from build123d import *

# Parameters (mm, degrees)
SKETCH1_W                = 65
SKETCH1_H                = 51.3
BOSS_EXTRUDE1_DEPTH      = 1.5
SKETCH2_W                = 17.929597568
SKETCH2_H                = 18
BOSS_EXTRUDE2_DEPTH      = 1
BOSS_EXTRUDE3_DEPTH      = 9
BOSS_EXTRUDE3_DEPTH_BACK = 11
SKETCH4_W                = 61
SKETCH4_H                = 3.022614149
SKETCH5_W                = 65
SKETCH5_H                = 51.3
BOSS_EXTRUDE4_DEPTH      = 1.5


with BuildPart() as part:
    # Sketch1 → Boss-Extrude1 (new body)
    with BuildSketch(Plane(origin=(0, 0, 0), x_dir=(1, 0, 0), z_dir=(0, 1, 0))):
        Rectangle(SKETCH1_W, SKETCH1_H)
    extrude(amount=BOSS_EXTRUDE1_DEPTH)

    # Sketch2 → Boss-Extrude2 (add)
    with BuildSketch(Plane(origin=(0, 1.5, 0), x_dir=(1, 0, 0), z_dir=(0, 1, 0))):
        with Locations((0, 11.65)):
            Rectangle(SKETCH2_W, SKETCH2_H)
        with Locations((0, -11.65)):
            Rectangle(SKETCH2_W, SKETCH2_H)
    extrude(amount=BOSS_EXTRUDE2_DEPTH)

    # Sketch4 → Boss-Extrude3 (add, two sides: drawn at the far end of the back side and taken through both)
    with BuildSketch(Plane.XZ.offset(-BOSS_EXTRUDE3_DEPTH_BACK)):
        with Locations((0, 22.138692926)):
            Rectangle(SKETCH4_W, SKETCH4_H)
        with Locations((0, -22.138692926)):
            Rectangle(SKETCH4_W, SKETCH4_H)
    extrude(amount=BOSS_EXTRUDE3_DEPTH + BOSS_EXTRUDE3_DEPTH_BACK)

    # Sketch5 → Boss-Extrude4 (add)
    with BuildSketch(Plane.XZ.offset(9)):
        Rectangle(SKETCH5_W, SKETCH5_H)
    extrude(amount=BOSS_EXTRUDE4_DEPTH)


solid = part.part
Geometry check sheet. Reference: the model listing, model coordinates, mm. A direction names the side the tool comes from. Round coordinates to 2 decimals unless told otherwise and drop trailing zeros. Loops run counter-clockwise (first coordinate to the right, second up) from the corner with the lowest first, then second, coordinate; pieces in that order, holes last. Notation, with made-up numbers: (86, -9) -> (102, -9) arc R18 cw to (102, 13) -> close; hole circle Ø4 at (-3.75, 73.25). An arc over 180 degrees is marked (long way). Answer as a JSON object with one key per item and string values. Group by question number.
Item 1: Cross-section at B-B, the plane z = 0. Record the cut outline in (x, y), plus the area to 3 significant figures.
Item 2: Cross-section at D-D, the plane z = 22.5. Record the cut outline in (x, y), plus the area to 3 significant figures.
Item 3: Thickness scan on line 1 along Y through (x, z) = (-23, -6.5); line 2 along Z through (x, y) = (7, 7.5); line 3 along Y through (x, z) = (5, -11.5). Record the ranges inside material, lowest first.
Item 4: Set-up check for faces 1 (the face through (-30.5, 6, -22)), 2 (the face through (0, 2.5, -12)), 3 (the face through (30.5, 6, -22)), 4 (the face through (0, -4, 20.627)), 5 (the face through (0, -4, -23.65)): record each of +Z, -Z, +X, -X, +Y, -Y from which the full face is reachable in a straight line by a thin tool's end or side.
Item 5: Cross-section at A-A, the plane x = -4.5. Record the cut outline in (y, z), plus the area to 3 significant figures.
Item 6: Cross-section at C-C, the plane y = -5.25. Record the cut outline in (x, z), plus the area to 3 significant figures.
Item 7: Depth check by flat-ended pin: pin 1 Ø3 at (x, y) = (-8, 8.5) entering from +Z; pin 2 Ø3.5 at (y, z) = (-3, 22) entering from -X; pin 3 Ø0.5 at (y, z) = (2, -10.5) entering from -X. Enter the tip coordinate at first touch or a pass-through.
Item 8: Release check for a two-part mould opening along Y. For faces 6 (the face through (32.5, -10, 0)), 7 (the face through (0, 11, -22)), 8 (the face through (-30.5, -4, 22)) record: pulls with the +Y half, pulls with the -Y half, needs draft (parallel to the pull), parting line crosses it, or undercut.
Determined:
{
 "1": {"outline": "(-32.5, -10.5) -> (32.5, -10.5) -> (32.5, -9) -> (-32.5, -9) -> close; (-32.5, 0) -> (32.5, 0) -> (32.5, 1.5) -> (-32.5, 1.5) -> close", "area": "195 mm²"},
 "2": {"outline": "(-32.5, -10.5) -> (32.5, -10.5) -> (32.5, -9) -> (30.5, -9) -> (30.5, 0) -> (32.5, 0) -> (32.5, 1.5) -> (30.5, 1.5) -> (30.5, 11) -> (-30.5, 11) -> (-30.5, 1.5) -> (-32.5, 1.5) -> (-32.5, 0) -> (-30.5, 0) -> (-30.5, -9) -> (-32.5, -9) -> close", "area": "1,320 mm²"},
 "3": {"line 1": "y = -10.5 to -9, 0 to 1.5", "line 2": "z = -23.65 to -20.63, 20.63 to 23.65", "line 3": "y = -10.5 to -9, 0 to 2.5"},
 "4": {"face 1": "+Z, -Z, -X, +Y", "face 2": "+X, -X, +Y", "face 3": "+Z, -Z, +X, +Y", "face 4": "+X, -X", "face 5": "-Z, +X, -X"},
 "5": {"outline": "(-10.5, -25.65) -> (-9, -25.65) -> (-9, -23.65) -> (0, -23.65) -> (0, -25.65) -> (1.5, -25.65) -> (1.5, -23.65) -> (11, -23.65) -> (11, -20.63) -> (2.5, -20.63) -> (2.5, -2.65) -> (1.5, -2.65) -> (1.5, 2.65) -> (2.5, 2.65) -> (2.5, 20.63) -> (11, 20.63) -> (11, 23.65) -> (1.5, 23.65) -> (1.5, 25.65) -> (0, 25.65) -> (0, 23.65) -> (-9, 23.65) -> (-9, 25.65) -> (-10.5, 25.65) -> close; hole (-9, -20.63) -> (0, -20.63) -> (0, 20.63) -> (-9, 20.63) -> close", "area": "302 mm²"},
 "6": {"outline": "(-30.5, -23.65) -> (30.5, -23.65) -> (30.5, -20.63) -> (-30.5, -20.63) -> close; (-30.5, 20.63) -> (30.5, 20.63) -> (30.5, 23.65) -> (-30.5, 23.65) -> close", "area": "369 mm²"},
 "7": {"pin 1": "stops at z = 23.65", "pin 2": "stops at x = -30.5", "pin 3": "stops at x = -8.96"},
 "8": {"face 6": "needs draft", "face 7": "pulls with the +Y half", "face 8": "undercut"}
}
